from build123d import *

# Parameters (mm, degrees)
BOSS_EXTRUDE1_DEPTH     = 15
CUT_EXTRUDE1_DEPTH      = 32.064449134
CUT_EXTRUDE1_DEPTH_BACK = 32.064449134
SKETCH2_W               = 7.5
SKETCH2_H               = 10
SKETCH3_R               = 1.5
CUT_EXTRUDE2_DEPTH      = 32.064449134


with BuildPart() as part:
    # Sketch1 → Boss-Extrude1 (new body)
    with BuildSketch(Plane(origin=(0, 0, 0), x_dir=(1, 0, 0), z_dir=(0, 1, 0))):
        with BuildLine():
            Line((1, 1.732050808), (1, 14))
            Line((1, 14), (19, 14))
            Line((19, 14), (19, 1.732050808))
            ThreePointArc((19, 1.732050808), (20, -2), (21, 1.732050808))
            Line((21, 1.732050808), (21, 16))
            Line((21, 16), (-1, 16))
            Line((-1, 16), (-1, 1.732050808))
            ThreePointArc((-1, 1.732050808), (0, -2), (1, 1.732050808))
        make_face()
    extrude(amount=BOSS_EXTRUDE1_DEPTH)

    # Sketch2 → Cut-Extrude1 (cut, two sides: drawn at the far end of the back side and taken through both)
    with BuildSketch(Plane(origin=(0, 0, 0), x_dir=(0, 0, -1), z_dir=(1, 0, 0)).offset(-CUT_EXTRUDE1_DEPTH_BACK)):
        with Locations((1.75, 7.5)):
            Rectangle(SKETCH2_W, SKETCH2_H)
    extrude(amount=CUT_EXTRUDE1_DEPTH + CUT_EXTRUDE1_DEPTH_BACK, mode=Mode.SUBTRACT)

    # Sketch3 → Cut-Extrude2 (cut, through all)
    with BuildSketch(Plane(origin=(0, 15, 0), x_dir=(1, 0, 0), z_dir=(0, 1, 0))):
        with Locations(Location((0, 0, 0), (0, 0, 270))):
            Circle(SKETCH3_R)
        with Locations(Location((20, 0, 0), (0, 0, 270))):
            Circle(SKETCH3_R)
    extrude(amount=-CUT_EXTRUDE2_DEPTH, mode=Mode.SUBTRACT)


solid = part.part
Verification items for the finished model (mm, model axes). A direction names the side the tool comes from. Give positions to 0.01 mm unless a question says otherwise; leave off trailing zeros. Order: outer loops, then holes, each group sorted by start corner. A loop starts at its lowest first (then second) coordinate and runs counter-clockwise, first axis right, second up. Notation, with made-up numbers: M -33,70.25 L -21,70.25 A8 ccw -21,77.25 Z; hole C -40,11 d1. An arc over 180 degrees is marked long. Use one line per item in the form item = value. Start each with the question number.
Q1. Section check A-A (z = -4). Enter the section's corners in (x, y).
Q2. Section check C-C (z = 0). Count the separate pieces of the cut face and the enclosed holes in it, then the cut area to 3 significant figures.
Q3. Mould release check, pull along Y, two halves, no side actions. Record for faces 5 (the flat face through (20, 7, -5.5)), 6 (the flat face through (21, 7, -10)): +Y half, -Y half, draft (parallel to the pull), parting line (faces both ways), or undercut.
Q4. Section check D-D (z = -7). Enter the section's corners in (x, y), then the cut area to 3 significant figures.
Q5. Go/stop test with flat-tipped pins: pin 1 Ø3 at (y, z) = (5, -5.5) entering from +X; pin 2 Ø6 at (y, z) = (8.5, -3) entering from -X; pin 3 Ø1.6 at (x, y) = (0, 10) entering from +Z; pin 4 Ø2.5 at (x, z) = (0, 0) entering from -Y. Record where each tip stops, or that it passes through.
Q6. Access from +Z, -Z, +X, -X, +Y, -Y to the whole of each face (thin tool, end or side, straight path). Record for faces 1 (the flat face through (-1, 7, -11)), 2 (the flat face through (10, 7, -16)), 3 (the flat face through (19, 7, -9)), 4 (the flat face through (0, 7, -5.5)).
Q7. Scan lines: line 1 along X through (y, z) = (1, 0); line 2 along X through (y, z) = (13.25, -10.75); line 3 along Z through (x, y) = (13.5, 4.75). Record each from-to range of solid material in increasing order. Write a range as [from, to].
Q8. Section check B-B (x = 20). Enter the section's corners in (y, z), then the cut area to 3 significant figures.
Evaluation:
q1.outline = M -1,0 L 1,0 L 1,2.5 L -1,2.5 Z; M -1,12.5 L 1,12.5 L 1,15 L -1,15 Z; M 19,0 L 21,0 L 21,2.5 L 19,2.5 Z; M 19,12.5 L 21,12.5 L 21,15 L 19,15 Z
q2.separate_pieces = 8
q2.enclosed_holes = 0
q2.area = 10.0 mm2
q3.face_5 = undercut
q3.face_6 = draft
q4.outline = M -1,0 L 1,0 L 1,15 L -1,15 Z; M 19,0 L 21,0 L 21,15 L 19,15 Z
q4.area = 60.0 mm2
q5.pin_1 = 21
q5.pin_2 = -1
q5.pin_3 = -5.5
q5.pin_4 = through
q6.face_1 = -Z, -X, +Y, -Y
q6.face_2 = -Z, +X, -X, +Y, -Y
q6.face_3 = +Y, -Y
q6.face_4 = +Z, +X, -X
q7.line_1 = [-2, -1.5], [1.5, 2], [18, 18.5], [21.5, 22]
q7.line_2 = [-1, 1], [19, 21]
q7.line_3 = [-16, -14]
q8.outline = M 0,-16 L 15,-16 L 15,-1.5 L 12.5,-1.5 L 12.5,-5.5 L 2.5,-5.5 L 2.5,-1.5 L 0,-1.5 Z; M 0,1.5 L 2.5,1.5 L 2.5,2 L 0,2 Z; M 12.5,1.5 L 15,1.5 L 15,2 L 12.5,2 Z
q8.area = 180 mm2
